Check sheet for the modelled part. Datum: model origin and axes. Units: mm. A direction names the side the tool comes from. Coordinates: 2 decimals unless noted, no trailing zeros. Order: outer loops, then holes, each group sorted by start corner. A loop starts at its lowest first (then second) coordinate and runs counter-clockwise, first axis right, second up. Notation, with made-up numbers: (30.25, 37.5) -> (68.25, 37.5) arc R28 ccw to (68.25, 74.5) -> close; hole circle Ø1 at (62.25, -20). An arc over 180 degrees is marked (long way). Put each result on its own line as item: value. Start each with the question number.
```python
from build123d import *

# Parameters (mm, degrees)
CROQUIS1_W              = 133
CROQUIS1_H              = 76
SALIENTE_EXTRUIR1_DEPTH = 10
CROQUIS2_W              = 110
CROQUIS2_H              = 65
CORTAR_EXTRUIR1_DEPTH   = 2
CROQUIS3_W              = 2
CROQUIS3_H              = 56
SALIENTE_EXTRUIR6_DEPTH = 3.5
CROQUIS4_W              = 2.5
CROQUIS4_H              = 56
CORTAR_EXTRUIR2_DEPTH   = 1.1
CROQUIS5_W              = 2.5
CROQUIS5_H              = 56
CORTAR_EXTRUIR3_DEPTH   = 1.1
CROQUIS6_W              = 2.5
CROQUIS6_H              = 56
CORTAR_EXTRUIR4_DEPTH   = 1.1
CROQUIS7_W              = 2.5
CROQUIS7_H              = 56
CORTAR_EXTRUIR5_DEPTH   = 1.1


with BuildPart() as part:
    # Croquis1 → Saliente-Extruir1 (new body)
    with BuildSketch(Plane.XY):
        with Locations((0, 38)):
            Rectangle(CROQUIS1_W, CROQUIS1_H)
    extrude(amount=SALIENTE_EXTRUIR1_DEPTH)

    # Croquis2 → Cortar-Extruir1 (cut)
    with BuildSketch(Plane(origin=(0, 0, 0), x_dir=(-1, 0, 0), z_dir=(0, 0, -1))):
        with Locations((0, 38)):
            Rectangle(CROQUIS2_W, CROQUIS2_H)
    extrude(amount=-CORTAR_EXTRUIR1_DEPTH, mode=Mode.SUBTRACT)

    # Croquis3 → Saliente-Extruir6 (add)
    with BuildSketch(Plane.XY.offset(10)):
        Polygon((-26, 68), (-26, 66), (-24, 66), (-16, 66), (-14, 66), (-14, 68), align=None)
        with Locations((-25, 38)):
            Rectangle(CROQUIS3_W, CROQUIS3_H)
        with Locations((-15, 38)):
            Rectangle(CROQUIS3_W, CROQUIS3_H)
        with Locations((15, 38)):
            Rectangle(CROQUIS3_W, CROQUIS3_H)
        Polygon((14, 66), (16, 66), (24, 66), (26, 66), (26, 68), (14, 68), align=None)
        with Locations((25, 38)):
            Rectangle(CROQUIS3_W, CROQUIS3_H)
    extrude(amount=SALIENTE_EXTRUIR6_DEPTH)

    # Croquis4 → Cortar-Extruir2 (cut)
    with BuildSketch(Plane(origin=(-24, 0, 0), x_dir=(0, 0, -1), z_dir=(1, 0, 0))):
        with Locations((-11.25, 38)):
            Rectangle(CROQUIS4_W, CROQUIS4_H)
    extrude(amount=-CORTAR_EXTRUIR2_DEPTH, mode=Mode.SUBTRACT)

    # Croquis5 → Cortar-Extruir3 (cut)
    with BuildSketch(Plane.ZY.offset(16)):
        with Locations((11.25, 38)):
            Rectangle(CROQUIS5_W, CROQUIS5_H)
    extrude(amount=-CORTAR_EXTRUIR3_DEPTH, mode=Mode.SUBTRACT)

    # Croquis6 → Cortar-Extruir4 (cut)
    with BuildSketch(Plane(origin=(16, 0, 0), x_dir=(0, 0, -1), z_dir=(1, 0, 0))):
        with Locations((-11.25, 38)):
            Rectangle(CROQUIS6_W, CROQUIS6_H)
    extrude(amount=-CORTAR_EXTRUIR4_DEPTH, mode=Mode.SUBTRACT)

    # Croquis7 → Cortar-Extruir5 (cut)
    with BuildSketch(Plane.ZY.offset(-24)):
        with Locations((11.25, 38)):
            Rectangle(CROQUIS7_W, CROQUIS7_H)
    extrude(amount=-CORTAR_EXTRUIR5_DEPTH, mode=Mode.SUBTRACT)


solid = part.part
```
1) Scan lines: line 1 along X through (y, z) = (53.5, 11); line 2 along Y through (x, z) = (-11.5, 1); line 3 along Z through (x, y) = (-21, 65). Record each from-to range of solid material in increasing order. Write a range as [from, to].
2) Access from +Z, -Z, +X, -X, +Y, -Y to the whole of each face (thin tool, end or side, straight path). Record for faces 1 (the flat face through (-14, 39, 12)), 2 (the flat face through (20, 68, 12)), 3 (the flat face through (26, 39, 12)).
3) Gauge pin test, flat ends, axial feed: pin 1 (2 mm diameter, centred on x = 42.5, z = 11.5, fed in from -Y); pin 2 (1.8 mm diameter, centred on x = 20.5, z = 11.5, fed in from +Y); pin 3 (3 mm diameter, centred on y = 34, z = 12, fed in from +X); pin 4 (1 mm diameter, centred on x = -19, z = 11.5, fed in from -Y). Record the tip position at first contact, or that the pin passes through.
4) Mould release check, pull along Z, two halves, no side actions. Record for faces 4 (the flat face through (14, 39, 12)), 5 (the flat face through (-14.9, 38, 11)), 6 (the flat face through (1, 38, 2)), 7 (the flat face through (15, 39, 13.5)): +Z half, -Z half, draft (parallel to the pull), parting line (faces both ways), or undercut.
5) Sectioned sample at C-C (x = -18). Record the boundary of the cut face in (y, z), plus the area to 3 significant figures.
6) Sectioned sample at D-D (x = -3). Record the boundary of the cut face in (y, z).
7) Sectioned sample at B-B (z = 11.25). Record the boundary of the cut face in (x, y), plus the area to 3 significant figures.
Entries:
1. line 1: x = [-26, -25.1], [-14.9, -14], [14, 14.9], [25.1, 26]
1. line 2: y = [0, 5.5], [70.5, 76]
1. line 3: z = [2, 10]
2. face 1: +Z, +Y, -Y
2. face 2: +Z, +X, -X, +Y
2. face 3: +Z, +X, +Y, -Y
3. pin 1: passes through
3. pin 2: stops at y = 68
3. pin 3: stops at x = 26
3. pin 4: stops at y = 66
4. face 4: draft
4. face 5: undercut
4. face 6: -Z half
4. face 7: +Z half
5. outline: (0, 0) -> (5.5, 0) -> (5.5, 2) -> (70.5, 2) -> (70.5, 0) -> (76, 0) -> (76, 10) -> (68, 10) -> (68, 13.5) -> (66, 13.5) -> (66, 10) -> (0, 10) -> close
5. area: 637 mm2
6. outline: (0, 0) -> (5.5, 0) -> (5.5, 2) -> (70.5, 2) -> (70.5, 0) -> (76, 0) -> (76, 10) -> (0, 10) -> close
7. outline: (-26, 10) -> (-25.1, 10) -> (-25.1, 66) -> (-14.9, 66) -> (-14.9, 10) -> (-14, 10) -> (-14, 68) -> (-26, 68) -> close; (14, 10) -> (14.9, 10) -> (14.9, 66) -> (25.1, 66) -> (25.1, 10) -> (26, 10) -> (26, 68) -> (14, 68) -> close
7. area: 250 mm2
